Source: CAD feature listing. Evaluate the final solid. Frame: model axes, mm. Round coordinates to 2 decimals unless told otherwise and drop trailing zeros. Write item = value, one per line.
from build123d import *

# Parameters (mm, degrees)
SKIZZE1_W                                   = 300
SKIZZE1_H                                   = 300
AUFSATZ_LINEAR_AUSTRAGEN1_DEPTH             = 4
VERRUNDUNG1_R                               = 17
FORMSENKUNG_F_R_M6_SENKSCHRAUBE_MIT_2_COUNT = 2
FORMSENKUNG_F_R_M6_SENKSCHRAUBE_MIT_2_PITCH = 280
FORMSENKUNG_F_R_M6_SENKSCHRAUBE_MIT_3_COUNT = 2
FORMSENKUNG_F_R_M6_SENKSCHRAUBE_MIT_3_PITCH = 395.979797464
FORMSENKUNG_F_R_M6_SENKSCHRAUBE_MIT_4_COUNT = 2
FORMSENKUNG_F_R_M6_SENKSCHRAUBE_MIT_4_PITCH = 280


with BuildPart() as part:
    # Skizze1 → Aufsatz-Linear austragen1 (new body)
    with BuildSketch(Plane(origin=(0, 0, 0), x_dir=(1, 0, 0), z_dir=(0, 1, 0))):
        with Locations((150, 150)):
            Rectangle(SKIZZE1_W, SKIZZE1_H)
    extrude(amount=AUFSATZ_LINEAR_AUSTRAGEN1_DEPTH)

    # Verrundung1
    verrundung1_edges = [part.edges().sort_by_distance(p)[0] for p in [
        (0, 2, -300),
        (300, 2, -300),
        (300, 2, 0),
        (0, 2, 0),
    ]]
    fillet(verrundung1_edges, radius=VERRUNDUNG1_R)

    # Skizze2 → Formsenkung für M6 Senkschraube mit Schlitz/Kreuzschlitz1 (revolve, cut)
    with BuildSketch(Plane(origin=(290, 4, -10), x_dir=(0, 0, 1), z_dir=(1, 0, 0))):
        Polygon((0, 0), (0, 4), (3.2, 4), (3.2, 3.1), (6.3, 0), align=None)
    formsenkung_f_r_m6_senkschraube_mit_schl = revolve(axis=Axis((290, 10.35, -10), (0, -1, 0)), mode=Mode.SUBTRACT)

    # Formsenkung f_r M6 Senkschraube mit  2: Formsenkung für M6 Senkschraube mit Schlitz/Kreuzschlitz1 ×2
    with Locations(*[(-i * FORMSENKUNG_F_R_M6_SENKSCHRAUBE_MIT_2_PITCH, 0, 0) for i in range(1, FORMSENKUNG_F_R_M6_SENKSCHRAUBE_MIT_2_COUNT)]):
        add(formsenkung_f_r_m6_senkschraube_mit_schl, mode=Mode.SUBTRACT)

    # Formsenkung f_r M6 Senkschraube mit  3: Formsenkung für M6 Senkschraube mit Schlitz/Kreuzschlitz1 ×2
    with Locations(*[Vector(-0.7071067811865475, 0, -0.7071067811865476) * (i * FORMSENKUNG_F_R_M6_SENKSCHRAUBE_MIT_3_PITCH) for i in range(1, FORMSENKUNG_F_R_M6_SENKSCHRAUBE_MIT_3_COUNT)]):
        add(formsenkung_f_r_m6_senkschraube_mit_schl, mode=Mode.SUBTRACT)

    # Formsenkung f_r M6 Senkschraube mit  4: Formsenkung für M6 Senkschraube mit Schlitz/Kreuzschlitz1 ×2
    with Locations(*[(0, 0, -i * FORMSENKUNG_F_R_M6_SENKSCHRAUBE_MIT_4_PITCH) for i in range(1, FORMSENKUNG_F_R_M6_SENKSCHRAUBE_MIT_4_COUNT)]):
        add(formsenkung_f_r_m6_senkschraube_mit_schl, mode=Mode.SUBTRACT)


solid = part.part
1. Contact query for flat-ended pins moving along their axis: pin 1 Ø6 at (x, z) = (290, -10) entering from -Y (1 decimal); pin 2 Ø10 at (x, z) = (10, -290) entering from +Y. Output: stop coordinate, or through.
Evaluation:
pin_1 = through
pin_2 = 2.7
2. Mould query, pull axis X, two halves, no side actions, for faces 1 (the face through (4.85, 2.03, -5.11)), 2 (the face through (291.226, 0.456, -287.044)), 3 (the face through (294.89, 2.03, -4.85)). Classes: released by +X, released by -X, zero draft, split by the parting line, or undercut.
Evaluation:
face_1 = released by -X
face_2 = undercut
face_3 = released by +X
3. Line query: probe 1 along X at (y, z) = (0.7, -10); probe 2 along Z at (x, y) = (290, 0.2). Output: solid intervals per line, ascending. Write a range as from..to.
Evaluation:
probe_1 = 1.51..6.8, 13.2..286.8, 293.2..298.49
probe_2 = -298.49..-293.2, -286.8..-13.2, -6.8..-1.51
